```python
from build123d import *

# Parameters (mm, degrees)
SKETCH1_W                         = 38.1
SKETCH1_H                         = 12.7
BOSS_EXTRUDE1_DEPTH               = 88.9
F_1_4_20_TAPPED_HOLE1_AT_2_COUNT  = 2
F_1_4_20_TAPPED_HOLE1_AT_2_PITCH  = 20.32
F_1_64_TAPPED_HOLE1_D             = 1.5113
F_1_4_20_TAPPED_HOLE3_D           = 5.1054
F_1_4_20_TAPPED_HOLE3_DEPTH       = 13.97
F_1_4_20_TAPPED_HOLE3_CSINK_D     = 6.3754
F_1_4_20_TAPPED_HOLE3_CSINK_ANGLE = 90
F_1_4_20_TAPPED_HOLE3_TIP         = 1.533816902


with BuildPart() as part:
    # Sketch1 → Boss-Extrude1 (new body)
    with BuildSketch(Plane.XY):
        Rectangle(SKETCH1_W, SKETCH1_H)
    extrude(amount=-BOSS_EXTRUDE1_DEPTH)

    # Sketch4 → 1/4-20 Tapped Hole1 (revolve, cut)
    with BuildSketch(Plane(origin=(-10.16, 0, 0), x_dir=(0, -1, 0), z_dir=(1, 0, 0))):
        Polygon((0, 0), (0, 14.233816902), (2.5527, 12.7), (2.5527, 0.635), (3.1877, 0), align=None)
    f_1_4_20_tapped_hole1 = revolve(axis=Axis((-10.16, 0, 6.35), (0, 0, -1)), mode=Mode.SUBTRACT)

    # 1/4-20 Tapped Hole1 at 2: 1/4-20 Tapped Hole1 ×2
    with Locations(*[(i * F_1_4_20_TAPPED_HOLE1_AT_2_PITCH, 0, 0) for i in range(1, F_1_4_20_TAPPED_HOLE1_AT_2_COUNT)]):
        add(f_1_4_20_tapped_hole1, mode=Mode.SUBTRACT)

    # Mirror1: 1/4-20 Tapped Hole1 across plane
    add(f_1_4_20_tapped_hole1.mirror(Plane.XY.offset(-44.45)), mode=Mode.SUBTRACT)

    # Mirror1 copy 1 sketch → Mirror1 copy 1 (revolve, cut)
    with BuildSketch(Plane(origin=(10.16, 0, -88.9), x_dir=(0, -1, 0), z_dir=(1, 0, 0))):
        Polygon((0, 0), (0, -14.233816902), (2.5527, -12.7), (2.5527, -0.635), (3.1877, 0), align=None)
    revolve(axis=Axis((10.16, 0, -95.25), (0, 0, -1)), mode=Mode.SUBTRACT)

    # #1-64 Tapped Hole1 (through all)
    with Locations(Plane(origin=(0, 6.35, -82.55), x_dir=(0, 0, 1), z_dir=(0, 1, 0))):
        with Locations((0, 0), (76.2, 0)):
            Hole(F_1_64_TAPPED_HOLE1_D / 2)

    # 1/4-20 Tapped Hole3
    with Locations(Plane.ZY.offset(19.05)):
        with Locations((-69.85, 0), (-19.05, 0)):
            CounterSinkHole(F_1_4_20_TAPPED_HOLE3_D / 2, F_1_4_20_TAPPED_HOLE3_CSINK_D / 2, depth=F_1_4_20_TAPPED_HOLE3_DEPTH, counter_sink_angle=F_1_4_20_TAPPED_HOLE3_CSINK_ANGLE)
            with Locations((0, 0, -(F_1_4_20_TAPPED_HOLE3_DEPTH + F_1_4_20_TAPPED_HOLE3_TIP / 2))):  # 118° drill point
                Cone(0, F_1_4_20_TAPPED_HOLE3_D / 2, F_1_4_20_TAPPED_HOLE3_TIP, mode=Mode.SUBTRACT)


solid = part.part
```
Design review of the part built by this model. Coordinates are the model's own, in mm. A direction names the side the tool comes from. Coordinates: 2 decimals unless noted, no trailing zeros. Order: outer loops, then holes, each group sorted by start corner. A loop starts at its lowest first (then second) coordinate and runs counter-clockwise, first axis right, second up. Notation, with made-up numbers: (-26.5, 45.25) -> (3.5, 45.25) arc R18 ccw to (3.5, 64.25) -> close; hole circle Ø8 at (-21.5, 28.25). An arc over 180 degrees is marked (long way). One line per item, written item: value. Start each with the question number.
Q1. Tool access review of faces 4 (the cylindrical face through (-11.654, 1.725, -17.169)), 5 (the cylindrical face through (7.63, 0.33, -82.32)), 6 (the cylindrical face through (7.63, 0.33, -6.58)): name each direction out of +Z, -Z, +X, -X, +Y, -Y from which nothing blocks a thin tool from reaching the whole face with its end or side.
Q2. Insertion check: pin 1 Ø4 at (x, y) = (-10.16, 0) entering from +Z; pin 2 Ø3 at (x, y) = (10.16, 0) entering from -Z; pin 3 Ø0.9 at (x, z) = (0, -6.35) entering from -Y; pin 4 Ø4 at (y, z) = (0, -19.05) entering from -X. Each pin has a flat end and moves straight along its axis. Give the tip position at first contact, or say it passes through.
Q3. Take a section at B-B, the plane y = -1.5. Give the number of separate pieces and of enclosed holes in the cut face, then the cut area to 3 significant figures.
Q4. Mouldability with a two-part tool opening along Y and no side actions: class faces 1 (the conical face through (-3.813, -0.17, -69.44)), 2 (the flat face through (0, -6.35, -44)), 3 (the cylindrical face through (0.033, -0.089, -5.595)) as pulls with the +Y half, pulls with the -Y half, needs draft (parallel to the pull), parting line crosses it, or undercut.
Q5. Take a section at A-A, the plane z = -8.5. State the section outline as (x, y) points.
Q6. For probe 1 along X at (y, z) = (0, -80); probe 2 along Y at (x, z) = (-10.16, -82); probe 3 along X at (y, z) = (1.25, -82.55), list the stretches that pass through material, from the lowest coordinate up.
Values follow:
1. face 4: -X
1. face 5: -Z
1. face 6: +Z
2. pin 1: stops at z = -13.03
2. pin 2: stops at z = -75.57
2. pin 3: passes through
2. pin 4: stops at x = -4.75
3. separate pieces: 1
3. enclosed holes: 2
3. area: 3,050 mm2
4. face 1: undercut
4. face 2: pulls with the -Y half
4. face 3: needs draft
5. outline: (-19.05, -6.35) -> (19.05, -6.35) -> (19.05, 6.35) -> (-19.05, 6.35) -> close; hole circle Ø5.11 at (-10.16, 0); hole circle Ø5.11 at (10.16, 0)
6. probe 1: x = -19.05 to -12.71, -7.61 to 7.61, 12.71 to 19.05
6. probe 2: y = -6.35 to -2.55, 2.55 to 6.35
6. probe 3: x = -19.05 to -12.39, -7.93 to -0.76, 0.76 to 7.93, 12.39 to 19.05
